from build123d import *

# Parameters (mm, degrees)
BOSS_EXTRUDE1_DEPTH = 1


with BuildPart() as part:
    # Sketch2 → Boss-Extrude1 (new body)
    with BuildSketch(Plane(origin=(0, 0, 0), x_dir=(1, 0, 0), z_dir=(0, 1, 0))):
        with BuildLine():
            Line((-10.5, -21.25), (10.5, -21.25))
            ThreePointArc((10.5, -21.25), (18.101397898, -18.101397898), (21.25, -10.5))
            Line((21.25, -10.5), (21.25, 10.5))
            ThreePointArc((21.25, 10.5), (18.101397898, 18.101397898), (10.5, 21.25))
            Line((10.5, 21.25), (-10.5, 21.25))
            ThreePointArc((-10.5, 21.25), (-18.101397898, 18.101397898), (-21.25, 10.5))
            Line((-21.25, 10.5), (-21.25, -10.5))
            ThreePointArc((-21.25, -10.5), (-18.101397898, -18.101397898), (-10.5, -21.25))
        make_face()
    extrude(amount=BOSS_EXTRUDE1_DEPTH)

    # Sweep3: sweep along a path in Sketch3
    with BuildLine(Plane(origin=(0, 1, 0), x_dir=(1, 0, 0), z_dir=(0, 1, 0))) as sweep3_path:
        Line((10.25, 19), (-10.25, 19))
        ThreePointArc((-10.25, 19), (-16.437184335, 16.437184335), (-19, 10.25))
        Line((-19, 10.25), (-19, -10.25))
        ThreePointArc((-19, -10.25), (-16.437184335, -16.437184335), (-10.25, -19))
        Line((-10.25, -19), (10.25, -19))
        ThreePointArc((10.25, -19), (16.437184335, -16.437184335), (19, -10.25))
        Line((19, -10.25), (19, 10.25))
        ThreePointArc((19, 10.25), (16.437184335, 16.437184335), (10.25, 19))
    # Sketch11 → Sweep3 (sweep)
    with BuildSketch(Plane.XY):
        with BuildLine():
            Line((-14, 1), (-19, 1))
            Line((-19, 1), (-19, 2.5))
            Line((-19, 2.5), (-19.26, 2.5))
            ThreePointArc((-19.26, 2.5), (-19.606482323, 2.643517677), (-19.75, 2.99))
            Line((-19.75, 2.99), (-19.75, 3.01))
            ThreePointArc((-19.75, 3.01), (-19.606482323, 3.356482323), (-19.26, 3.5))
            Line((-19.26, 3.5), (-19, 3.5))
            Line((-19, 3.5), (-19, 4.01))
            ThreePointArc((-19, 4.01), (-18.856482323, 4.356482323), (-18.51, 4.5))
            Line((-18.51, 4.5), (-14.49, 4.5))
            ThreePointArc((-14.49, 4.5), (-14.143517677, 4.356482323), (-14, 4.01))
            Line((-14, 4.01), (-14, 1))
        make_face()
    sweep(path=sweep3_path.line)


solid = part.part
Model file for the job. Use its own axes, mm. A direction names the side the tool comes from. Give positions to 0.01 mm unless a question says otherwise; leave off trailing zeros. Order: outer loops, then holes, each group sorted by start corner. A loop starts at its lowest first (then second) coordinate and runs counter-clockwise, first axis right, second up. Notation, with made-up numbers: M -14,-20.5 L 10,-20.5 A30 ccw 10,7.5 Z; hole C -19.5,31 d10. An arc over 180 degrees is marked long. Write item = value, one per line.
Q1. Drill centre lines: line 1 (Z direction, x = 8, y = 1.05); line 2 (Y direction, x = 13, z = 9). Where is each one in solid material? Low to high. Write a range as [from, to].
Derived:
line_1 = [-19, -14], [14, 19]
line_2 = [0, 1]
Q2. Two-plate mould, pull along X, no slides. Class faces 5 (the cylindrical face through (16.369, 1.74, 16.505)), 6 (the cylindrical face through (12.931, 2.526, -12.872)), 7 (the flat face through (0, 1, -21)): pulls with the +X half, pulls with the -X half, needs draft (parallel to the pull), parting line crosses it, or undercut.
Derived:
face_5 = pulls with the +X half
face_6 = undercut
face_7 = needs draft
Q3. Tool access for faces 1 (the cylindrical face through (-16.369, 3.751, -16.505)), 2 (the cylindrical face through (16.369, 3.751, 16.505)), 3 (the cylindrical face through (16.505, 1.74, -16.369)), 4 (the flat face through (0, 2, 14)): list every direction of +Z, -Z, +X, -X, +Y, -Y with a clear straight run to the whole face (end or side of a thin tool).
Derived:
face_1 = -Z, -X, +Y
face_2 = +Z, +X, +Y
face_3 = -Z, +X
face_4 = +Y
Q4. Flat gauge pins, fed straight in: pin 1 (0.8 mm diameter, centred on x = 1.5, y = 1.5, fed in from -Z); pin 2 (2.5 mm diameter, centred on y = 3, z = 4, fed in from +X); pin 3 (1.5 mm diameter, centred on x = 17, y = 1.5, fed in from -Z). Where does each tip first touch, or does it go through?
Derived:
pin_1 = -19
pin_2 = 19.75
pin_3 = -19.46
Q5. Cut at A-A, the plane y = 1.5. List the corners of the cut face in (x, z), then the cut area to 3 significant figures.
Derived:
outline = M -19,-10.25 A8.75 ccw -10.25,-19 L 10.25,-19 A8.75 ccw 19,-10.25 L 19,10.25 A8.75 ccw 10.25,19 L -10.25,19 A8.75 ccw -19,10.25 Z; hole M -14,-10.25 A3.75 ccw -10.25,-14 L 10.25,-14 A3.75 ccw 14,-10.25 L 14,10.25 A3.75 ccw 10.25,14 L -10.25,14 A3.75 ccw -14,10.25 Z
area = 606 mm2
